from build123d import *

# Parameters (mm, degrees)
EXTRUDE_1_DEPTH     = 47.2
CUT_EXTRUDE_2_REACH = 77.476
CUT_EXTRUDE_START   = -3
SKETCH_2_W          = 66
SKETCH_2_H          = 43.2
CUT_EXTRUDE_3_REACH = 66.937
SKETCH_3_R          = 1.6
SKETCH_3_R_2        = 6.6
CUT_EXTRUDE_4_REACH = 74.476
SKETCH_4_R          = 1.6
FILLET_1_R          = 1
SKETCH_5_W          = 15
SKETCH_5_H          = 10
EXTRUDE_2_DEPTH     = 2


with BuildPart() as part:
    # 草图1 → 凸台-拉伸1 (new body)
    with BuildSketch(Plane(origin=(0, 0, 0), x_dir=(1, 0, 0), z_dir=(0, 1, 0))):
        with BuildLine():
            Line((33, 30), (12.193267422, -6.879260831))
            ThreePointArc((12.193267422, -6.879260831), (0, -14), (-12.193267422, -6.879260831))
            Line((-12.193267422, -6.879260831), (-33, 30))
            Line((-33, 30), (33, 30))
        make_face()
    extrude(amount=EXTRUDE_1_DEPTH)

    # 草图2 → 切除-拉伸2 (cut, up to next)
    with BuildSketch(Plane(origin=(0, 0, -30), x_dir=(-1, 0, 0), z_dir=(0, 0, -1)).offset(CUT_EXTRUDE_START), mode=Mode.PRIVATE) as cut_extrude_2_sk1:
        with Locations((0, 23.6)):
            Rectangle(SKETCH_2_W, SKETCH_2_H)
    cut_extrude_2_tool1 = extrude(cut_extrude_2_sk1.sketch, amount=-CUT_EXTRUDE_2_REACH, mode=Mode.PRIVATE) & part.part
    add(cut_extrude_2_tool1.solids().sort_by_distance((0, 23.6, -27))[0], mode=Mode.SUBTRACT)

    # 切除-拉伸3: up to this face of the body (flat: up to its plane)
    cut_extrude_3_end = Plane(part.part.faces().sort_by_distance((0, 0, -12.723672626))[0])
    # 草图3 → 切除-拉伸3 (cut, up to the picked face)
    with BuildSketch(Plane(origin=(0, 47.2, 0), x_dir=(1, 0, 0), z_dir=(0, 1, 0)), mode=Mode.PRIVATE) as cut_extrude_3_sk1:
        with Locations(Location((-8.227241336, -4.75, 0), (0, 0, 90))):
            Circle(SKETCH_3_R)
    cut_extrude_3_tool1 = split(extrude(cut_extrude_3_sk1.sketch, amount=-CUT_EXTRUDE_3_REACH, mode=Mode.PRIVATE), bisect_by=cut_extrude_3_end, keep=Keep.BOTH, mode=Mode.PRIVATE)
    # 草图3 → 切除-拉伸3 (cut, up to the picked face)
    with BuildSketch(Plane(origin=(0, 47.2, 0), x_dir=(1, 0, 0), z_dir=(0, 1, 0)), mode=Mode.PRIVATE) as cut_extrude_3_sk2:
        with Locations(Location((8.227241336, -4.75, 0), (0, 0, 90))):
            Circle(SKETCH_3_R)
    cut_extrude_3_tool2 = split(extrude(cut_extrude_3_sk2.sketch, amount=-CUT_EXTRUDE_3_REACH, mode=Mode.PRIVATE), bisect_by=cut_extrude_3_end, keep=Keep.BOTH, mode=Mode.PRIVATE)
    # 草图3 → 切除-拉伸3 (cut, up to the picked face)
    with BuildSketch(Plane(origin=(0, 47.2, 0), x_dir=(1, 0, 0), z_dir=(0, 1, 0)), mode=Mode.PRIVATE) as cut_extrude_3_sk3:
        with Locations(Location((0, 0, 0), (0, 0, 90))):
            Circle(SKETCH_3_R_2)
    cut_extrude_3_tool3 = split(extrude(cut_extrude_3_sk3.sketch, amount=-CUT_EXTRUDE_3_REACH, mode=Mode.PRIVATE), bisect_by=cut_extrude_3_end, keep=Keep.BOTH, mode=Mode.PRIVATE)
    # 草图3 → 切除-拉伸3 (cut, up to the picked face)
    with BuildSketch(Plane(origin=(0, 47.2, 0), x_dir=(1, 0, 0), z_dir=(0, 1, 0)), mode=Mode.PRIVATE) as cut_extrude_3_sk4:
        with Locations(Location((0, 9.5, 0), (0, 0, 90))):
            Circle(SKETCH_3_R)
    cut_extrude_3_tool4 = split(extrude(cut_extrude_3_sk4.sketch, amount=-CUT_EXTRUDE_3_REACH, mode=Mode.PRIVATE), bisect_by=cut_extrude_3_end, keep=Keep.BOTH, mode=Mode.PRIVATE)
    add(cut_extrude_3_tool1.solids().sort_by(Axis((-8.227241, 47.2, 4.75), (0, -1, 0)))[0], mode=Mode.SUBTRACT)
    add(cut_extrude_3_tool2.solids().sort_by(Axis((8.227241, 47.2, 4.75), (0, -1, 0)))[0], mode=Mode.SUBTRACT)
    add(cut_extrude_3_tool3.solids().sort_by(Axis((0, 47.2, 0), (0, -1, 0)))[0], mode=Mode.SUBTRACT)
    add(cut_extrude_3_tool4.solids().sort_by(Axis((0, 47.2, -9.5), (0, -1, 0)))[0], mode=Mode.SUBTRACT)

    # 草图4 → 切除-拉伸4 (cut, up to next)
    with BuildSketch(Plane(origin=(0, 0, -30), x_dir=(-1, 0, 0), z_dir=(0, 0, -1)), mode=Mode.PRIVATE) as cut_extrude_4_sk1:
        with Locations((-27.5, 41.1)):
            Circle(SKETCH_4_R)
    cut_extrude_4_tool1 = extrude(cut_extrude_4_sk1.sketch, amount=-CUT_EXTRUDE_4_REACH, mode=Mode.PRIVATE) & part.part
    # 草图4 → 切除-拉伸4 (cut, up to next)
    with BuildSketch(Plane(origin=(0, 0, -30), x_dir=(-1, 0, 0), z_dir=(0, 0, -1)), mode=Mode.PRIVATE) as cut_extrude_4_sk2:
        with Locations((27.5, 41.1)):
            Circle(SKETCH_4_R)
    cut_extrude_4_tool2 = extrude(cut_extrude_4_sk2.sketch, amount=-CUT_EXTRUDE_4_REACH, mode=Mode.PRIVATE) & part.part
    # 草图4 → 切除-拉伸4 (cut, up to next)
    with BuildSketch(Plane(origin=(0, 0, -30), x_dir=(-1, 0, 0), z_dir=(0, 0, -1)), mode=Mode.PRIVATE) as cut_extrude_4_sk3:
        with Locations((27.5, 6.1)):
            Circle(SKETCH_4_R)
    cut_extrude_4_tool3 = extrude(cut_extrude_4_sk3.sketch, amount=-CUT_EXTRUDE_4_REACH, mode=Mode.PRIVATE) & part.part
    # 草图4 → 切除-拉伸4 (cut, up to next)
    with BuildSketch(Plane(origin=(0, 0, -30), x_dir=(-1, 0, 0), z_dir=(0, 0, -1)), mode=Mode.PRIVATE) as cut_extrude_4_sk4:
        with Locations((-27.5, 6.1)):
            Circle(SKETCH_4_R)
    cut_extrude_4_tool4 = extrude(cut_extrude_4_sk4.sketch, amount=-CUT_EXTRUDE_4_REACH, mode=Mode.PRIVATE) & part.part
    add(cut_extrude_4_tool1.solids().sort_by_distance((27.5, 41.1, -30))[0], mode=Mode.SUBTRACT)
    add(cut_extrude_4_tool2.solids().sort_by_distance((-27.5, 41.1, -30))[0], mode=Mode.SUBTRACT)
    add(cut_extrude_4_tool3.solids().sort_by_distance((-27.5, 6.1, -30))[0], mode=Mode.SUBTRACT)
    add(cut_extrude_4_tool4.solids().sort_by_distance((27.5, 6.1, -30))[0], mode=Mode.SUBTRACT)

    # 圆角1
    fillet_1_edges = [part.edges().sort_by_distance(p)[0] for p in [
        (0, 47.2, -30),
        (0, 0, -30),
        (-33, 23.6, -30),
        (33, 23.6, -30),
    ]]
    fillet(fillet_1_edges, radius=FILLET_1_R)

    # 草图5 → 凸台-拉伸2 (add)
    with BuildSketch(Plane.XY.offset(-27)):
        with Locations((23.807444446, 33.7)):
            Rectangle(SKETCH_5_W, SKETCH_5_H)
        with Locations((-23.807444446, 13.5)):
            Rectangle(SKETCH_5_W, SKETCH_5_H)
    extrude(amount=EXTRUDE_2_DEPTH)


solid = part.part
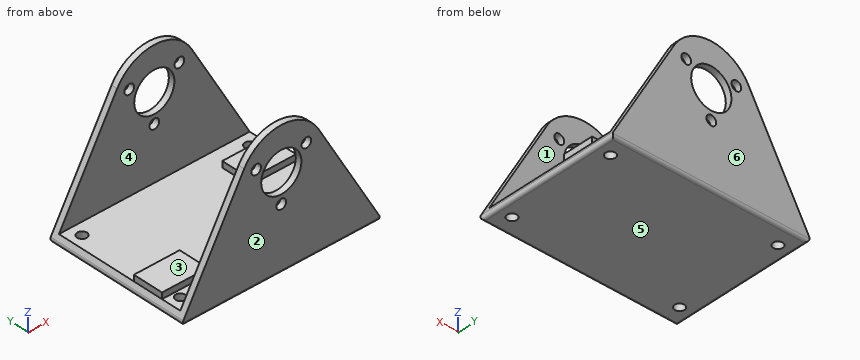
Read the model definition and answer for the solid it produces. Units are mm, in the model's axes. Face numbers are marked on the shaded views. A direction names the side the tool comes from. Coordinates: 2 decimals unless noted, no trailing zeros. Loops run counter-clockwise (first coordinate to the right, second up) from the corner with the lowest first, then second, coordinate; pieces in that order, holes last. Notation, with made-up numbers: (0, 87) -> (21, 87) arc R26 ccw to (21, 102) -> close; hole circle Ø9 at (19.25, 81.5). An arc over 180 degrees is marked (long way). Write item = value, one per line. Start each with the question number.
1) The part is cut by section D-D, the plane x = 27.5. Determine the outline of the cut face in (y, z).
2) For the marked faces 1 and 2, determine the directions among +Z, -Z, +X, -X, +Y, -Y from which every point of the face is accessible in a straight line to the end or side of a thin tool.
3) The part is cut by section C-C, the plane z = 0. Determine the outline of the cut face in (x, y), plus the area to 3 significant figures.
4) The part is cut by section A-A, the plane x = 0. Determine the outline of the cut face in (y, z), plus the area to 3 significant figures.
5) The mould has two halves that part along Y. Classify the marked faces 3, 4, 5 and 6: pulls with the +Y half, pulls with the -Y half, needs draft (parallel to the pull), parting line crosses it, or undercut.
6) Find the intervals of material crossed by L1, parallel to Y at x = 27.5, z = -27.6; L2, parallel to Y at x = -8.5, z = -13; L3, parallel to X at y = 0.6, z = 4.75, in increasing order. Write a range as from..to.
7) The part is cut by section B-B, the plane y = 41.1. Determine the outline of the cut face in (x, z), plus the area to 3 significant figures.
8) Given P1, Ø3, axis at x = 21, y = 34.5, coming from the +Z side; P2, Ø0.6, axis at y = 36, z = -26.5, coming from the +X side; P3, Ø2.5, axis at x = 27.5, y = 6.1, coming from the -Z side; P4, Ø0.6, axis at y = 16, z = -25.5, coming from the +X side, each flat-ended and moving along its own axis, determine where each tip first touches the part or whether it passes through.
Result:
q1.outline = (0, -29) arc R1 ccw to (1, -30) -> (4.5, -30) -> (4.5, -27) -> (2, -27) -> (2, -20.25) -> (0, -20.25) -> close; (7.7, -30) -> (39.5, -30) -> (39.5, -27) -> (38.7, -27) -> (38.7, -25) -> (28.7, -25) -> (28.7, -27) -> (7.7, -27) -> close; (42.7, -30) -> (46.2, -30) arc R1 ccw to (47.2, -29) -> (47.2, -20.25) -> (45.2, -20.25) -> (45.2, -27) -> (42.7, -27) -> close
q2.face_1 = +Z, +X, -X
q2.face_2 = +Z, -Z, +X, -X, -Y
q3.outline = (-16.07, 0) -> (-6.6, 0) -> (-6.6, 2) -> (-16.07, 2) -> close; (-16.07, 45.2) -> (-6.6, 45.2) -> (-6.6, 47.2) -> (-16.07, 47.2) -> close; (6.6, 0) -> (16.07, 0) -> (16.07, 2) -> (6.6, 2) -> close; (6.6, 45.2) -> (16.07, 45.2) -> (16.07, 47.2) -> (6.6, 47.2) -> close
q3.area = 75.8 mm²
q4.outline = (0, -29) arc R1 ccw to (1, -30) -> (46.2, -30) arc R1 ccw to (47.2, -29) -> (47.2, -11.1) -> (45.2, -11.1) -> (45.2, -27) -> (2, -27) -> (2, -11.1) -> (0, -11.1) -> close; (0, -7.9) -> (2, -7.9) -> (2, -6.6) -> (0, -6.6) -> close; (0, 6.6) -> (2, 6.6) -> (2, 14) -> (0, 14) -> close; (45.2, -7.9) -> (47.2, -7.9) -> (47.2, -6.6) -> (45.2, -6.6) -> close; (45.2, 6.6) -> (47.2, 6.6) -> (47.2, 14) -> (45.2, 14) -> close
q4.area = 240 mm²
q5.face_3 = undercut
q5.face_4 = undercut
q5.face_5 = needs draft
q5.face_6 = pulls with the +Y half
q6.L1 = 0..4.5, 7.7..39.5, 42.7..47.2
q6.L2 = 0..2, 45.2..47.2
q6.L3 = -13.39..-9.83, -6.63..-4.58, 4.58..6.63, 9.83..13.39
q7.outline = (-32.16, -28.51) arc R1 ccw to (-31.29, -30) -> (-29.1, -30) -> (-29.1, -27) -> (-31.31, -27) -> close; (-25.9, -30) -> (25.9, -30) -> (25.9, -27) -> (-25.9, -27) -> close; (29.1, -30) -> (31.29, -30) arc R1 ccw to (32.16, -28.51) -> (31.31, -27) -> (29.1, -27) -> close
q7.area = 172 mm²
q8.P1 = -25
q8.P2 = 31.31
q8.P3 = through
q8.P4 = -16.31
